from build123d import *

# Parameters (mm, degrees)
SKETCH_1_W          = 30.5
SKETCH_1_H          = 12
EXTRUDE_1_DEPTH     = 18
SKETCH_2_W          = 30.5
SKETCH_2_H          = 12
CUT_EXTRUDE_2_DEPTH = 6.2
SKETCH_3_R          = 2
SKETCH_3_W          = 4
SKETCH_3_H          = 1
CUT_EXTRUDE_3_DEPTH = 11.5
CUT_EXTRUDE_4_DEPTH = 8
SKETCH_5_W          = 3.964363922
SKETCH_5_H          = 1
CUT_EXTRUDE_6_DEPTH = 7
SKETCH_6_W          = 3.964363922
SKETCH_6_H          = 6
CUT_EXTRUDE_7_DEPTH = 26.822712871
FILLET_1_R          = 2
FILLET_2_R          = 2
FILLET_3_R          = 1
SKETCH_7_W          = 17.4
SKETCH_7_H          = 5.750693342
CUT_EXTRUDE_8_DEPTH = 10.5
SKETCH_9_R          = 0.5
CUT_EXTRUDE_9_DEPTH = 8
SKETCH_8_R          = 0.25
EXTRUDE_2_DEPTH     = 3


with BuildPart() as part:
    # 草图1 → 凸台-拉伸1 (new body)
    with BuildSketch(Plane(origin=(0, 0, 0), x_dir=(1, 0, 0), z_dir=(0, 1, 0))):
        Rectangle(SKETCH_1_W, SKETCH_1_H)
    extrude(amount=EXTRUDE_1_DEPTH)

    # 草图2 → 切除-拉伸2 (cut)
    with BuildSketch(Plane(origin=(0, 18, 0), x_dir=(1, 0, 0), z_dir=(0, 1, 0))):
        Rectangle(SKETCH_2_W, SKETCH_2_H)
        with BuildLine():
            Line((-6.556600226, 3), (6.556600226, 3))
            ThreePointArc((6.556600226, 3), (6.924541369, 2.838554744), (7.054873105, 2.45847726))
            Line((7.054873105, 2.45847726), (6.638206438, -2.54152274))
            ThreePointArc((6.638206438, -2.54152274), (6.478488304, -2.867941143), (6.139933559, -3))
            Line((6.139933559, -3), (-6.139933559, -3))
            ThreePointArc((-6.139933559, -3), (-6.478488304, -2.867941143), (-6.638206438, -2.54152274))
            Line((-6.638206438, -2.54152274), (-7.054873105, 2.45847726))
            ThreePointArc((-7.054873105, 2.45847726), (-6.924541369, 2.838554744), (-6.556600226, 3))
        make_face(mode=Mode.SUBTRACT)
    extrude(amount=-CUT_EXTRUDE_2_DEPTH, mode=Mode.SUBTRACT)

    # 草图3 → 切除-拉伸3 (cut)
    with BuildSketch(Plane(origin=(0, 11.8, 0), x_dir=(1, 0, 0), z_dir=(0, 1, 0))):
        with Locations(Location((12.25, 0, 0), (0, 0, 270))):
            Circle(SKETCH_3_R)
        with Locations(Location((-12.25, 0, 0), (0, 0, 90))):
            Circle(SKETCH_3_R)
        with Locations((12.25, -5.5)):
            Rectangle(SKETCH_3_W, SKETCH_3_H)
        with Locations((-12.25, -5.5)):
            Rectangle(SKETCH_3_W, SKETCH_3_H)
    extrude(amount=-CUT_EXTRUDE_3_DEPTH, mode=Mode.SUBTRACT)

    # 草图4 → 切除-拉伸4 (cut)
    with BuildSketch(Plane.XZ):
        Polygon((8.5, -4.6), (8.5, 3.5), (15.25, 3.5), (15.25, -4.6), (15.25, -6), (-15.25, -6), (-15.25, 3.5), (-8.5, 3.5), (-8.5, -4.6), align=None)
    extrude(amount=-CUT_EXTRUDE_4_DEPTH, mode=Mode.SUBTRACT)

    # 草图5 → 切除-拉伸6 (cut)
    with BuildSketch(Plane.XZ):
        with Locations((12.267818039, 4)):
            Rectangle(SKETCH_5_W, SKETCH_5_H)
        with Locations((-12.267818039, 4)):
            Rectangle(SKETCH_5_W, SKETCH_5_H)
    extrude(amount=-CUT_EXTRUDE_6_DEPTH, mode=Mode.SUBTRACT)

    # 草图6 → 切除-拉伸7 (cut, through all)
    with BuildSketch(Plane(origin=(0, 0, 4.5), x_dir=(-1, 0, 0), z_dir=(0, 0, -1))):
        with Locations((12.267818039, 4)):
            Rectangle(SKETCH_6_W, SKETCH_6_H)
    cut_extrude_7 = extrude(amount=-CUT_EXTRUDE_7_DEPTH, mode=Mode.SUBTRACT)

    # 圆角1
    # the kernel refuses this fillet: 2 mm, written as the material it adds along each edge
    with BuildSketch(Plane(origin=(-14.25, 1, 4.5), x_dir=(0, 1, 0), z_dir=(0, 0, 1)), Plane(origin=(-10.285636078, 1, 4.5), x_dir=(-1, 0, 0), z_dir=(0, 0, 1))) as fillet_1_piece_1:
        with BuildLine():
            CenterArc((FILLET_1_R, -FILLET_1_R), FILLET_1_R, 90, 90)
            Line((0, -FILLET_1_R), (0, 0))
            Line((0, 0), (FILLET_1_R, 0))
        make_face()
    extrude(amount=0.5)
    with BuildSketch(Plane(origin=(-14.25, 7, 3.5), x_dir=(0, -1, 0), z_dir=(0, 0, 1))) as fillet_1_piece_2:
        with BuildLine():
            CenterArc((FILLET_1_R, FILLET_1_R), FILLET_1_R, 180, 90)
            Line((0, FILLET_1_R), (0, 0))
            Line((0, 0), (FILLET_1_R, 0))
        make_face()
    extrude(amount=1.5)
    with BuildSketch(Plane(origin=(-10.285636078, 7, 3.5), x_dir=(0, -1, 0), z_dir=(0, 0, 1))) as fillet_1_piece_3:
        with BuildLine():
            CenterArc((FILLET_1_R, -FILLET_1_R), FILLET_1_R, 90, 90)
            Line((0, -FILLET_1_R), (0, 0))
            Line((0, 0), (FILLET_1_R, 0))
        make_face()
    extrude(amount=1.5)

    # 镜向1: 切除-拉伸7 across plane
    add(cut_extrude_7.mirror(Plane(origin=(0, 0, 0), x_dir=(0, 0, 1), z_dir=(1, 0, 0))), mode=Mode.SUBTRACT)

    # 圆角2
    # the kernel refuses this fillet: 2 mm, written as the material it adds along each edge
    with BuildSketch(Plane(origin=(14.25, 1, 4.5), x_dir=(-1, 0, 0), z_dir=(0, 0, 1))) as fillet_2_piece_1:
        with BuildLine():
            CenterArc((FILLET_2_R, -FILLET_2_R), FILLET_2_R, 90, 90)
            Line((0, -FILLET_2_R), (0, 0))
            Line((0, 0), (FILLET_2_R, 0))
        make_face()
    extrude(amount=0.5)
    with BuildSketch(Plane(origin=(10.285636078, 1, 4.5), x_dir=(1, 0, 0), z_dir=(0, 0, 1))) as fillet_2_piece_2:
        with BuildLine():
            CenterArc((FILLET_2_R, FILLET_2_R), FILLET_2_R, 180, 90)
            Line((0, FILLET_2_R), (0, 0))
            Line((0, 0), (FILLET_2_R, 0))
        make_face()
    extrude(amount=0.5)
    with BuildSketch(Plane(origin=(10.285636078, 7, 3.5), x_dir=(1, 0, 0), z_dir=(0, 0, 1)), Plane(origin=(14.25, 7, 5), x_dir=(-1, 0, 0), z_dir=(0, 0, -1))) as fillet_2_piece_3:
        with BuildLine():
            CenterArc((FILLET_2_R, -FILLET_2_R), FILLET_2_R, 90, 90)
            Line((0, -FILLET_2_R), (0, 0))
            Line((0, 0), (FILLET_2_R, 0))
        make_face()
    extrude(amount=1.5)

    # 圆角3
    fillet_3_edges = [part.edges().sort_by_distance(p)[0] for p in [
        (-15.25, 9.9, -6),
        (15.25, 9.9, -6),
        (-8.5, 4, -4.6),
        (8.5, 4, -4.6),
    ]]
    fillet(fillet_3_edges, radius=FILLET_3_R)

    # 草图7 → 切除-拉伸8 (cut)
    with BuildSketch(Plane.XZ):
        with Locations((0, 7.875346671)):
            Rectangle(SKETCH_7_W, SKETCH_7_H)
    extrude(amount=-CUT_EXTRUDE_8_DEPTH, mode=Mode.SUBTRACT)

    # 草图9 → 切除-拉伸9 (cut)
    with BuildSketch(Plane(origin=(0, 18, 0), x_dir=(1, 0, 0), z_dir=(0, 1, 0))):
        with Locations(Location((0, 1.27, 0), (0, 0, 270))):
            Circle(SKETCH_9_R)
        with Locations(Location((2.54, 1.27, 0), (0, 0, 270))):
            Circle(SKETCH_9_R)
        with Locations(Location((5.08, 1.27, 0), (0, 0, 270))):
            Circle(SKETCH_9_R)
        with Locations(Location((-5.08, 1.27, 0), (0, 0, 90))):
            Circle(SKETCH_9_R)
        with Locations(Location((-2.54, 1.27, 0), (0, 0, 90))):
            Circle(SKETCH_9_R)
        with Locations(Location((-1.27, -1.27, 0), (0, 0, 270))):
            Circle(SKETCH_9_R)
        with Locations(Location((-3.81, -1.27, 0), (0, 0, 270))):
            Circle(SKETCH_9_R)
        with Locations(Location((3.81, -1.27, 0), (0, 0, 90))):
            Circle(SKETCH_9_R)
        with Locations(Location((1.27, -1.27, 0), (0, 0, 90))):
            Circle(SKETCH_9_R)
    extrude(amount=-CUT_EXTRUDE_9_DEPTH, mode=Mode.SUBTRACT)

    # 草图8 → 凸台-拉伸2 (add)
    with BuildSketch(Plane.XY.offset(5)):
        with Locations(Location((0, 1.27, 0), (0, 0, 180))):
            Circle(SKETCH_8_R)
        with Locations(Location((2.77, 1.27, 0), (0, 0, 180))):
            Circle(SKETCH_8_R)
        with Locations(Location((5.54, 1.27, 0), (0, 0, 180))):
            Circle(SKETCH_8_R)
        with Locations(Location((-5.54, 1.27, 0), (0, 0, 180))):
            Circle(SKETCH_8_R)
        with Locations(Location((-2.77, 1.27, 0), (0, 0, 180))):
            Circle(SKETCH_8_R)
        with Locations(Location((-1.385, 4.11, 0), (0, 0, 180))):
            Circle(SKETCH_8_R)
        with Locations(Location((1.385, 4.11, 0), (0, 0, 180))):
            Circle(SKETCH_8_R)
        with Locations(Location((-4.155, 4.11, 0), (0, 0, 180))):
            Circle(SKETCH_8_R)
        with Locations(Location((4.155, 4.11, 0), (0, 0, 180))):
            Circle(SKETCH_8_R)
    extrude(amount=EXTRUDE_2_DEPTH)


solid = part.part
Work out the finished part from the listing and answer in its coordinate system (mm). A direction names the side the tool comes from. Give positions to 0.01 mm unless a question says otherwise; leave off trailing zeros. Loops run counter-clockwise (first coordinate to the right, second up) from the corner with the lowest first, then second, coordinate; pieces in that order, holes last. Notation, with made-up numbers: (43, 61.25) - (77, 61.25) arc R12 ccw to (77, 83.25) - close; hole circle Ø8 at (28, 49.25). An arc over 180 degrees is marked (long way). Answer in a Markdown table with one row per item. Add a question column.
Q1. Each of these flat-tipped pins is pushed along its axis until it touches: P1, Ø4, axis at x = -2, z = 6, coming from the +Y side; P2, Ø1.9, axis at x = 0, y = 14, coming from the -Z side; P3, Ø4.5, axis at x = -12, y = 9, coming from the +Z side. Where does it stop, or does it pass through?
Q2. A tool of negligible diameter and unlimited length cuts with its end or side. For faces 1 (the cylindrical face through (8.199, 4.056, -4.315)), 2 (the cylindrical face through (-1.12, 14.056, 1.747)), 3 (the flat face through (-14.25, 4.5, 5)), from which of +Z, -Z, +X, -X, +Y, -Y can it reach the whole face along a straight path? Write none if from no direction.
Q3. Consider line 1 along X through (y, z) = (10.1, 0); line 2 along X through (y, z) = (5, 5.5); line 3 along Z through (x, y) = (3.81, 13). Determine where each line is inside the solid, lowest interval first.
Q4. The part is cut by section C-C (y = 13.5). State how many separate pieces and enclosed holes the cut face has, and give its area (3 significant figures).
Q5. The part is cut by section A-A (z = 0). Determine the outline of the cut face in (x, y), and give its area (3 significant figures).
Q6. The part is cut by section B-B (x = -13). Determine the outline of the cut face in (y, z).
Q7. The part is cut by section D-D (x = -8). Determine the outline of the cut face in (y, z).
Q8. Determine the mould class of faces 4 (the flat face through (-10, 6, 3.5)), 5 (the cylindrical face through (10.88, 6.42, 4.24)), 6 (the flat face through (-15.25, 8.4, 1.8)) for opening direction X: released by +X, released by -X, zero draft, split by the parting line, or undercut.
Solution:
| question | item | result |
|---|---|---|
| 1 | P1 | stops at y = 11.8 |
| 1 | P2 | stops at z = -3 |
| 1 | P3 | stops at z = 6 |
| 2 | face 1 | -Z, +X, -Y |
| 2 | face 2 | +Y |
| 2 | face 3 | none |
| 3 | line 1 | x = -15.25 to -14.25, -10.25 to 10.25, 14.25 to 15.25 |
| 3 | line 2 | x = -15.25 to -14.25, -10.25 to -8.7, 8.7 to 10.25, 14.25 to 15.25 |
| 3 | line 3 | z = -3 to 0.77, 1.77 to 3 |
| 4 | separate pieces | 1 |
| 4 | enclosed holes | 9 |
| 4 | area | 74.9 mm² |
| 5 | outline | (-15.25, 8) - (-14.25, 8) - (-14.25, 11.8) - (-15.25, 11.8) - close; (-10.25, 8) - (-8.5, 8) - (-8.5, 0) - (8.5, 0) - (8.5, 8) - (10.25, 8) - (10.25, 11.8) - (6.85, 11.8) - (6.85, 18) - (-6.85, 18) - (-6.85, 11.8) - (-10.25, 11.8) - close; (14.25, 8) - (15.25, 8) - (15.25, 11.8) - (14.25, 11.8) - close |
| 5 | area | 306 mm² |
| 6 | outline | (0, 4.5) - (1.15, 4.5) - (1.15, 5) - (0.3, 5) - (0.3, 6) - (0, 6) - close; (6.85, 3.5) - (8, 3.5) - (8, 1.85) - (11.8, 1.85) - (11.8, 5) - (6.85, 5) - close; (8, -6) - (11.8, -6) - (11.8, -1.85) - (8, -1.85) - close |
| 7 | outline | (0, -4.47) - (8, -4.47) - (8, -6) - (11.8, -6) - (11.8, 6) - (10.5, 6) - (10.5, 5) - (0, 5) - close |
| 8 | face 4 | zero draft |
| 8 | face 5 | undercut |
| 8 | face 6 | released by -X |
